Can you work these out from the model? Positions are in its coordinate system, mm. Give positions to 0.01 mm unless a question says otherwise; leave off trailing zeros. Loops run counter-clockwise (first coordinate to the right, second up) from the corner with the lowest first, then second, coordinate; pieces in that order, holes last. Notation, with made-up numbers: (5.5, -38.5) - (29.5, -38.5) arc R24 cw to (29.5, -24.5) - close; hole circle Ø10 at (48, 61). An arc over 180 degrees is marked (long way). Answer as a JSON object with one key per item and string values. Group by question number.
Item 1: Suppose I cut it at B-B on y = 1.25. Write out the boundary of the cut face in (x, z).
Item 2: Suppose I cut it at C-C on x = 4. Write out the boundary of the cut face in (y, z), and give its area (3 significant figures).
Item 3: Please list where this line runs through material, in increasing order: L1, parallel to Z at x = 5, y = 1.7.
Item 4: Suppose I cut it at A-A on x = 5. Write out the boundary of the cut face in (y, z).
from build123d import *

# Parameters (mm, degrees)
SKETCH001_R  = 0.25
PAD001_DEPTH = 3.5
SKETCH_W     = 7.5
SKETCH_H     = 4.6
PAD_DEPTH    = 10.5
FILLET_R     = 0.2


with BuildPart() as pad001:
    # Sketch001 → Pad001 (new body)
    with BuildSketch(Plane.XY.offset(0.5)):
        Circle(SKETCH001_R)
        with Locations((5, 0)):
            Circle(SKETCH001_R)
    extrude(amount=-PAD001_DEPTH)


with BuildPart() as obj1:
    # Sketch → Pad (new body)
    with BuildSketch(Plane.XY.offset(0.1)):
        with Locations((2.5, 0)):
            Rectangle(SKETCH_W, SKETCH_H)
    extrude(amount=PAD_DEPTH)

    # Fillet
    fillet_edges = [obj1.edges().sort_by_distance(p)[0] for p in [
        (6.25, -2.3, 5.35),
        (6.25, 2.3, 5.35),
        (-1.25, -2.3, 5.35),
        (-1.25, 2.3, 5.35),
    ]]
    fillet(fillet_edges, radius=FILLET_R)

    # obj1: union Pad001
    add(pad001.part)


solid = obj1.part
Worked out:
{
 "1": {"outline": "(-1.25, 0.1) - (6.25, 0.1) - (6.25, 10.6) - (-1.25, 10.6) - close"},
 "2": {"outline": "(-2.3, 0.1) - (2.3, 0.1) - (2.3, 10.6) - (-2.3, 10.6) - close", "area": "48.3 mm2"},
 "3": {"L1": "z = 0.1 to 10.6"},
 "4": {"outline": "(-2.3, 0.1) - (-0.25, 0.1) - (-0.25, -3) - (0.25, -3) - (0.25, 0.1) - (2.3, 0.1) - (2.3, 10.6) - (-2.3, 10.6) - close"}
}
